Read the model definition and answer for the solid it produces. Units are mm, in the model's axes. A direction names the side the tool comes from. Round coordinates to 2 decimals unless told otherwise and drop trailing zeros. Order: outer loops, then holes, each group sorted by start corner. A loop starts at its lowest first (then second) coordinate and runs counter-clockwise, first axis right, second up. Notation, with made-up numbers: M -20,72 L 24,72 A27 cw 24,100 Z; hole C 89.5,84 d8. An arc over 180 degrees is marked long. Answer as CSV lines item,"result".
Autodesk Inventor part; units mm, degrees
ref_plane "YZ Plane" through (0, 0, 0) normal (1, 0, 0) x (0, 1, 0)
ref_plane "XZ Plane" through (0, 0, 0) normal (0, 1, 0) x (-1, 0, 0)
ref_plane "XY Plane" through (0, 0, 0) normal (0, 0, 1) x (1, 0, 0)
sketch "Sketch1" plane through (0, 0, 0) normal (0, 1, 0) x (-1, 0, 0)
  line L0 (-38.5, 22) -> (38.5, 22)
  line L1 (38.5, 22) -> (38.5, -22)
  line L2 (38.5, -22) -> (-38.5, -22)
  line L3 (-38.5, -22) -> (-38.5, 22)
  line L4 (-38.5, 22) -> (38.5, -22) construction
  line L5 (38.5, 22) -> (-38.5, -22) construction
  line L6 (38.5, -22) -> (-38.5, -22)
  line L7 (-38.5, -22) -> (-38.5, 21)
  line L8 (38.5, 21) -> (38.5, -22)
  line L9 (-38, 24.5) -> (38, 24.5)
  line L10 (41, 21.5) -> (41, -21.5)
  line L11 (38, -24.5) -> (-38, -24.5)
  line L12 (-41, -21.5) -> (-41, 21.5)
  line L13 (-41, 24.5) -> (41, -24.5) construction
  line L14 (41, 24.5) -> (-41, -24.5) construction
  arc A0 (41, 21.5) -> (38, 24.5) centre (38, 21.5) ccw
  arc A1 (38, -24.5) -> (41, -21.5) centre (38, -21.5) ccw
  arc A2 (-41, -21.5) -> (-38, -24.5) centre (-38, -21.5) ccw
  arc A3 (-38, 24.5) -> (-41, 21.5) centre (-38, 21.5) ccw
  point P0 (0, 0)
  dimension "d0" = 77
  dimension "d1" = 44
  dimension "d3" = 82
  dimension "d4" = 49
  dimension "d5" = 3
extrude "Extrusion1" add sketch "Sketch1" along normal blind 2 contours L0 L1 L2 L3 | L9 A0 L10 A1 L11 A2 L12 A3
sketch "Sketch22" plane through (0, 2, 0) normal (0, 1, 0) x (1, 0, 0)
  line L0 (38, 24.5) -> (-38, 24.5)
  arc A0 (-38, 24.5) -> (-41, 21.5) centre (-38, 21.5) ccw
  line L1 (-41, 21.5) -> (-41, -21.5)
  arc A1 (-41, -21.5) -> (-38, -24.5) centre (-38, -21.5) ccw
  line L2 (-38, -24.5) -> (38, -24.5)
  arc A2 (38, -24.5) -> (41, -21.5) centre (38, -21.5) ccw
  line L3 (41, -21.5) -> (41, 21.5)
  arc A3 (41, 21.5) -> (38, 24.5) centre (38, 21.5) ccw
  line L4 (-38.5, -22) -> (38.5, -22)
  line L5 (38.5, -22) -> (38.5, 22)
  line L6 (38.5, 22) -> (-38.5, 22)
  line L7 (-38.5, 22) -> (-38.5, -22)
  point P0 (0, 0)
  dimension "d80" = 2.5
  dimension "d81" = 2.5
  dimension "d82" = 2.5
  dimension "d83" = 2.5
extrude "Extrusion18" add sketch "Sketch22" along normal blind 22
fillet "Fillet5" radius 1 4 edges at (-38.5, 13, -22) (-38.5, 13, 22) (38.5, 13, 22) (38.5, 13, -22)
sketch "Sketch23" plane through (0, 24, 0) normal (0, 1, 0) x (1, 0, 0)
  line L0 (-38.75, 23.25) -> (38.75, 23.25)
  line L1 (39.75, 22.25) -> (39.75, -22.25)
  line L2 (38.75, -23.25) -> (-38.75, -23.25)
  line L3 (-39.75, -22.25) -> (-39.75, 22.25)
  line L4 (-39.75, 23.25) -> (39.75, -23.25) construction
  line L5 (39.75, 23.25) -> (-39.75, -23.25) construction
  line L6 (41, -21.5) -> (41, 21.5)
  line L7 (-38, -24.5) -> (38, -24.5)
  line L8 (-38.5, -21) -> (-38.5, 21)
  line L9 (-37.5, 22) -> (37.5, 22)
  line L10 (38.5, 21) -> (38.5, -21)
  line L11 (37.5, -22) -> (-37.5, -22)
  arc A0 (-38.5, -21) -> (-37.5, -22) centre (-37.5, -21) ccw
  arc A1 (-37.5, 22) -> (-38.5, 21) centre (-37.5, 21) ccw
  arc A2 (38.5, 21) -> (37.5, 22) centre (37.5, 21) ccw
  arc A3 (37.5, -22) -> (38.5, -21) centre (37.5, -21) ccw
  arc A4 (38.75, -23.25) -> (39.75, -22.25) centre (38.75, -22.25) ccw
  arc A5 (39.75, 22.25) -> (38.75, 23.25) centre (38.75, 22.25) ccw
  arc A6 (-38.75, 23.25) -> (-39.75, 22.25) centre (-38.75, 22.25) ccw
  arc A7 (-39.75, -22.25) -> (-38.75, -23.25) centre (-38.75, -22.25) ccw
  point P0 (0, 0)
  dimension "d87" = 1.25
  dimension "d88" = 1.25
  dimension "d91" = 1
extrude "Extrusion19" cut sketch "Sketch23" against normal blind 1
properties part number "Ver 1"
Item 1: A cutting plane is placed at A-A, the plane y = 20. Determine the outline of the cut face in (x, z).
Ans:
outline,"M -41,-21.5 A3 ccw -38,-24.5 L 38,-24.5 A3 ccw 41,-21.5 L 41,21.5 A3 ccw 38,24.5 L -38,24.5 A3 ccw -41,21.5 Z; hole M -38.5,-21 A1 ccw -37.5,-22 L 37.5,-22 A1 ccw 38.5,-21 L 38.5,21 A1 ccw 37.5,22 L -37.5,22 A1 ccw -38.5,21 Z"
Item 2: Determine the mould class of faces 1 (the face through (-0.2, 23, -22.5)), 2 (the face through (-40.14, 11.83, -23.6)), 3 (the face through (1, 12, -24.5)), 4 (the face through (41, 12, 0)) for opening direction X: +X half, -X half, draft (parallel to the pull), parting line (faces both ways), or undercut.
Ans:
face 1,"undercut"
face 2,"-X half"
face 3,"draft"
face 4,"+X half"
Item 3: A tool of negligible diameter and unlimited length cuts with its end or side. For faces 5 (the face through (1, 0, 0)), 6 (the face through (-1, 12, 22)), from which of +Z, -Z, +X, -X, +Y, -Y can it reach the whole face along a straight path? Write none if from no direction.
Ans:
face 5,"+Z, -Z, +X, -X, -Y"
face 6,"+Y"
Item 4: A cutting plane is placed at B-B, the plane z = -9. Determine the outline of the cut face in (x, y).
Ans:
outline,"M -41,0 L 41,0 L 41,24 L 39.75,24 L 39.75,23 L 38.5,23 L 38.5,2 L -38.5,2 L -38.5,23 L -39.75,23 L -39.75,24 L -41,24 Z"
Item 5: A flat-ended cylindrical pin translates along its axis: pin 1 (1 mm diameter, centred on x = 20, z = 18.5, fed in from +Y). Find the tip coordinate at first contact, or state that the pin passes through.
Ans:
pin 1,"y = 2"
Item 6: A cutting plane is placed at C-C, the plane x = 31. Determine the outline of the cut face in (y, z).
Ans:
outline,"M 0,-24.5 L 24,-24.5 L 24,-23.25 L 23,-23.25 L 23,-22 L 2,-22 L 2,22 L 23,22 L 23,23.25 L 24,23.25 L 24,24.5 L 0,24.5 Z"
Item 7: Find the intervals of material crossed by probe 1 along X at (y, z) = (3.75, -6); probe 2 along Z at (x, y) = (3, 19); probe 3 along Y at (x, z) = (2, 12), in increasing order. Write a range as [from, to].
Ans:
probe 1,"[-41, -38.5], [38.5, 41]"
probe 2,"[-24.5, -22], [22, 24.5]"
probe 3,"[0, 2]"
